Build history of the part. All positions in model axes, mm. A direction names the side the tool comes from. Coordinates: 2 decimals unless noted, no trailing zeros. Loops run counter-clockwise (first coordinate to the right, second up) from the corner with the lowest first, then second, coordinate; pieces in that order, holes last.
Item 1: Drill centre lines: line 1 along X through (y, z) = (-3.5, 13.5); line 2 along Y through (x, z) = (104, -4); line 3 along X through (y, z) = (-7, 3). Where is each one in solid material? Low to high.
Item 2: Cut at A-A (y = 0). List the corners of the cut face in (x, z), and give its area (3 significant figures).
Item 3: Cut at D-D (z = 11). List the corners of the cut face in (x, y), and give its area (3 significant figures).
Item 4: Cut at C-C (x = 48). List the corners of the cut face in (y, z).
Item 5: Mould opens along Z. For faces 4 (the face through (114.535, 12.536, 0.325)), 5 (the face through (131.675, -3.966, -0.521)), 6 (the face through (114.54, 0.07, 15.5)), 7 (the face through (117, 7, 7)) say: released by +Z, released by -Z, zero draft, split by the parting line, or undercut.
Item 6: Flat gauge pins, fed straight in: pin 1 (2 mm diameter, centred on y = -6, z = -8, fed in from +X); pin 2 (3 mm diameter, centred on x = 124.5, z = 1, fed in from +Y); pin 3 (6 mm diameter, centred on x = 127.5, y = -5.5, fed in from -Z). Where does each tip first touch, or does it go through?
Item 7: 3-axis set-ups, long thin cutter, end or side, ignore diameter. For faces 1 (the face through (36.504, -15.368, -2.018)), 2 (the face through (118.014, -8.428, -1.107)), 3 (the face through (137, 3, 0)): which of +Z, -Z, +X, -X, +Y, -Y reach the whole face in a straight line?
Item 8: Cut at B-B (z = 0). List the corners of the cut face in (x, y), and give its area (3 significant figures).
from build123d import *

# Parameters (mm, degrees)
CUT_EXTRUDE1_DEPTH = 15
SKETCH3_R          = 1.5
CUT_EXTRUDE2_DEPTH = 5


with BuildPart() as part:
    # Sketch1 → Revolve1 (revolve)
    with BuildSketch(Plane.XY, mode=Mode.PRIVATE) as revolve1_sk:
        Polygon((0, 0), (0, 15.5), (72, 15.5), (72, 16), (117, 16), (117, 8.5), (119, 8.5), (119, 4), (144, 4), (144, 0), align=None)
    revolve(revolve1_sk.sketch.rotate(Axis((0, 0, 0), (1, 0, 0)), 90), axis=Axis((0, 0, 0), (1, 0, 0)))

    # Sketch2 → Cut-Extrude1 (cut)
    with BuildSketch(Plane(origin=(144, 0, 0), x_dir=(0, 0, -1), z_dir=(1, 0, 0))):
        with BuildLine():
            Line((-2.645751311, 3), (2.645751311, 3))
            ThreePointArc((2.645751311, 3), (0, 4), (-2.645751311, 3))
        make_face()
    extrude(amount=-CUT_EXTRUDE1_DEPTH, mode=Mode.SUBTRACT)

    # Sketch3 → Cut-Extrude2 (cut)
    with BuildSketch(Plane(origin=(117, 0, 0), x_dir=(0, 0, -1), z_dir=(1, 0, 0))):
        with Locations((0, 14)):
            Circle(SKETCH3_R)
        with Locations((14, 0)):
            Circle(SKETCH3_R)
        with Locations((0, -14)):
            Circle(SKETCH3_R)
        with Locations((-14, 0)):
            Circle(SKETCH3_R)
    extrude(amount=-CUT_EXTRUDE2_DEPTH, mode=Mode.SUBTRACT)


solid = part.part
Filled sheet:
1. line 1: x = 0 to 117
1. line 2: y = -15.49 to 15.49
1. line 3: x = 0 to 119
2. outline: (0, -15.5) - (72, -15.5) - (72, -16) - (117, -16) - (117, -15.5) - (112, -15.5) - (112, -12.5) - (117, -12.5) - (117, -8.5) - (119, -8.5) - (119, -4) - (144, -4) - (144, 4) - (119, 4) - (119, 8.5) - (117, 8.5) - (117, 12.5) - (112, 12.5) - (112, 15.5) - (117, 15.5) - (117, 16) - (72, 16) - (72, 15.5) - (0, 15.5) - close
2. area: 3,880 mm2
3. outline: (0, -10.92) - (72, -10.92) - (72, -11.62) - (117, -11.62) - (117, 11.62) - (72, 11.62) - (72, 10.92) - (0, 10.92) - close
3. area: 2,620 mm2
4. outline: circle Ø31 at (0, 0)
5. face 4: undercut
5. face 5: split by the parting line
5. face 6: undercut
5. face 7: zero draft
6. pin 1: stops at x = 117
6. pin 2: stops at y = 4
6. pin 3: stops at z = -3.12
7. face 1: -X
7. face 2: +X
7. face 3: +Z, -Z, +X, +Y
8. outline: (0, -15.5) - (72, -15.5) - (72, -16) - (117, -16) - (117, -15.5) - (112, -15.5) - (112, -12.5) - (117, -12.5) - (117, -8.5) - (119, -8.5) - (119, -4) - (144, -4) - (144, 3) - (129, 3) - (129, 4) - (119, 4) - (119, 8.5) - (117, 8.5) - (117, 12.5) - (112, 12.5) - (112, 15.5) - (117, 15.5) - (117, 16) - (72, 16) - (72, 15.5) - (0, 15.5) - close
8. area: 3,860 mm2
